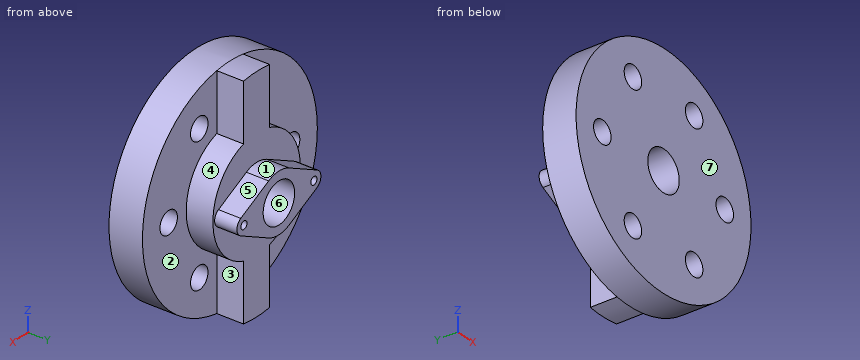
```python
from build123d import *
from build123d.topology import SkipClean

# Parameters (mm, degrees)
SKETCH1_R           = 50
BOSS_EXTRUDE1_DEPTH = 15
BOSS_EXTRUDE2_DEPTH = 12
SKETCH3_R           = 1.75
BOSS_EXTRUDE3_DEPTH = 10
HOLE1_D             = 18
HOLE2_D             = 10
CIRPATTERN1_COUNT   = 6


with BuildPart() as part:
    # Sketch1 → Boss-Extrude1 (new body)
    with BuildSketch(Plane(origin=(0, 0, 0), x_dir=(1, 0, 0), z_dir=(0, 1, 0))):
        with Locations(Location((0, 0, 0), (0, 0, 270))):
            Circle(SKETCH1_R)
    extrude(amount=BOSS_EXTRUDE1_DEPTH)

    # Sketch2 → Boss-Extrude2 (add)
    with SkipClean():  # the faces are left unmerged after this step: merging them gives an invalid solid
        with BuildSketch(Plane(origin=(0, 15, 0), x_dir=(1, 0, 0), z_dir=(0, 1, 0))):
            with BuildLine():
                Line((7.5, 49.434299833), (7.5, 23.848480035))
                ThreePointArc((7.5, 23.848480035), (25, 0), (7.5, -23.848480035))
                Line((7.5, -23.848480035), (7.5, -49.434299833))
                ThreePointArc((7.5, -49.434299833), (0, -50), (-7.5, -49.434299833))
                Line((-7.5, -49.434299833), (-7.5, -23.848480035))
                ThreePointArc((-7.5, -23.848480035), (-25, 0), (-7.5, 23.848480035))
                Line((-7.5, 23.848480035), (-7.5, 49.434299833))
                ThreePointArc((-7.5, 49.434299833), (0, 50), (7.5, 49.434299833))
            make_face()
        extrude(amount=BOSS_EXTRUDE2_DEPTH)

    # Sketch3 → Boss-Extrude3 (add)
    with SkipClean():  # the faces are left unmerged after this step: merging them gives an invalid solid
        with BuildSketch(Plane(origin=(0, 27, 0), x_dir=(1, 0, 0), z_dir=(0, 1, 0))):
            with BuildLine():
                Line((-21.8, 3.57211422), (-5.85, 11.609371215))
                ThreePointArc((-5.85, 11.609371215), (0, 13), (5.85, 11.609371215))
                Line((5.85, 11.609371215), (21.8, 3.57211422))
                ThreePointArc((21.8, 3.57211422), (24, 0), (21.8, -3.57211422))
                Line((21.8, -3.57211422), (5.85, -11.609371215))
                ThreePointArc((5.85, -11.609371215), (0, -13), (-5.85, -11.609371215))
                Line((-5.85, -11.609371215), (-21.8, -3.57211422))
                ThreePointArc((-21.8, -3.57211422), (-24, 0), (-21.8, 3.57211422))
            make_face()
            with Locations(Location((-20, 0, 0), (0, 0, 270))):
                Circle(SKETCH3_R, mode=Mode.SUBTRACT)
            with Locations(Location((20, 0, 0), (0, 0, 270))):
                Circle(SKETCH3_R, mode=Mode.SUBTRACT)
        extrude(amount=BOSS_EXTRUDE3_DEPTH)

    # Hole1 (through all)
    with Locations(Plane(origin=(0, 37, 0), x_dir=(1, 0, 0), z_dir=(0, 1, 0))):
        with Locations((0, 0)):
            Hole(HOLE1_D / 2)

    # Hole2 (through all)
    with Locations(Plane(origin=(0, 15, 0), x_dir=(1, 0, 0), z_dir=(0, 1, 0))):
        with Locations((35, 0)):
            hole2 = Hole(HOLE2_D / 2)

    # CirPattern1: Hole2 ×6 about axis
    with SkipClean():  # the faces are left unmerged after this step: merging them gives an invalid solid
        cirpattern1_axis = Axis((0, 0, 0), (0, 1, 0))
        for i in range(1, CIRPATTERN1_COUNT):
            add(hole2.rotate(cirpattern1_axis, i * 360 / CIRPATTERN1_COUNT), mode=Mode.SUBTRACT)


solid = part.part
```
Design review of the part built by this model. Coordinates are the model's own, in mm. Face numbers are marked on the shaded views. A direction names the side the tool comes from. Give positions to 0.01 mm unless a question says otherwise; leave off trailing zeros. Order: outer loops, then holes, each group sorted by start corner. A loop starts at its lowest first (then second) coordinate and runs counter-clockwise, first axis right, second up. Notation, with made-up numbers: (6, -36) - (31, -36) arc R12 cw to (31, -32) - close; hole circle Ø7 at (72, 54.25). An arc over 180 degrees is marked (long way). Use a Markdown table: item, result. Add a question column.
(1) Add section D-D on z = 29. Give the boundary of the cut face in (x, y), then the cut area to 3 significant figures.
(2) Clearance check with flat-ended pins moving along their axes: P1, Ø6, axis at x = -22.5, y = 27, coming from the +Z side; P2, Ø3, axis at x = -15, y = 32.5, coming from the +Z side; P3, Ø13, axis at y = 22.5, z = -31, coming from the -X side. State where each tip first meets the part, or that it passes through.
(3) Mouldability with a two-part tool opening along Z and no side actions: class the marked faces 4, 5, 6 and 7 as +Z half, -Z half, draft (parallel to the pull), parting line (faces both ways), or undercut.
(4) Machinability: for the marked faces 1, 2 and 3, which of the approach directions +Z, -Z, +X, -X, +Y, -Y give a long, thin tool a straight path to every point of the face, cutting with its end or side? Answer none if there is none.
(5) Add section C-C on x = 0. Give the boundary of the cut face in (y, z), then the cut area to 3 significant figures.
(6) Wall thickness on probe 1 along Z at (x, y) = (-17.5, 10.25); probe 2 along Z at (x, y) = (0, 25); probe 3 along Z at (x, y) = (17, 10): over which ranges is each line inside the solid? List them lowest first. Write a range as [from, to].
(7) Add section A-A on y = 21.5. Give the boundary of the cut face in (x, z), then the cut area to 3 significant figures.
(8) Add section B-B on z = 0. Give the number of separate pieces and of enclosed holes in the cut face, then the cut area to 3 significant figures.
Report:
| question | item | result |
|---|---|---|
| 1 | outline | (-40.73, 0) - (-22.33, 0) - (-22.33, 15) - (-40.73, 15) - close; (-12.67, 0) - (12.67, 0) - (12.67, 15) - (7.5, 15) - (7.5, 27) - (-7.5, 27) - (-7.5, 15) - (-12.67, 15) - close; (22.33, 0) - (40.73, 0) - (40.73, 15) - (22.33, 15) - close |
| 1 | area | 1,110 mm² |
| 2 | P1 | stops at z = 15.64 |
| 2 | P2 | stops at z = 7.75 |
| 2 | P3 | stops at x = -7.5 |
| 3 | face 4 | parting line |
| 3 | face 5 | +Z half |
| 3 | face 6 | undercut |
| 3 | face 7 | draft |
| 4 | face 1 | +Z, +Y |
| 4 | face 2 | +X, +Y |
| 4 | face 3 | -Z, +X, +Y |
| 5 | outline | (0, -50) - (27, -50) - (27, -13) - (37, -13) - (37, -9) - (0, -9) - close; (0, 9) - (37, 9) - (37, 13) - (27, 13) - (27, 50) - (0, 50) - close |
| 5 | area | 2,290 mm² |
| 6 | probe 1 | z = [-46.84, -35.31], [-25.31, 25.31], [35.31, 46.84] |
| 6 | probe 2 | z = [-50, -9], [9, 50] |
| 6 | probe 3 | z = [-47.02, -35.29], [-25.34, 25.34], [35.29, 47.02] |
| 7 | outline | (-7.5, -49.43) arc R50 ccw to (7.5, -49.43) - (7.5, -23.85) arc R25 ccw to (7.5, 23.85) - (7.5, 49.43) arc R50 ccw to (-7.5, 49.43) - (-7.5, 23.85) arc R25 ccw to (-7.5, -23.85) - close; hole circle Ø18 at (0, 0) |
| 7 | area | 2,460 mm² |
| 8 | separate pieces | 4 |
| 8 | enclosed holes | 0 |
| 8 | area | 1,540 mm² |
